from build123d import *

# Parameters (mm, degrees)
SKETCH_R     = 5.5
PAD_DEPTH    = 2
PAD001_DEPTH = 3.6


with BuildPart() as part:
    # Sketch → Pad (new body)
    with BuildSketch(Plane.XY):
        Circle(SKETCH_R)
    extrude(amount=PAD_DEPTH)

    # Sketch001 (on Face3 of Pad) → Pad001 (join)
    with BuildSketch(Plane.XY.offset(2)):
        with BuildLine():
            ThreePointArc((3.122117, 3.720795), (-2.7, 0), (3.122117, -3.720795))
            Line((3.122117, -3.720795), (3.400681, -4.322658))
            ThreePointArc((3.400681, 4.322658), (-5.5, 0), (3.400681, -4.322658))
            Line((3.122117, 3.720795), (3.400681, 4.322658))
        make_face()
    extrude(amount=PAD001_DEPTH)


solid = part.part
Model file for the job. Use its own axes, mm. Coordinates: 2 decimals unless noted, no trailing zeros. Loops run counter-clockwise (first coordinate to the right, second up) from the corner with the lowest first, then second, coordinate; pieces in that order, holes last. Notation, with made-up numbers: (35, -0.5) -> (80, -0.5) arc R35 ccw to (80, 33.5) -> close; hole circle Ø1 at (-11, 59). An arc over 180 degrees is marked (long way). Use one line per item in the form item = value. Start each with the question number.
(1) Probe probe 1 along Z at (x, y) = (-2.5, -0.5); probe 2 along Y at (x, z) = (1.25, 4.4); probe 3 along Y at (x, z) = (1.4, 4.7). List the from-to ranges inside material, lowest first. Write a range as from..to.
(2) Flat gauge pins, fed straight in: pin 1 (4 mm diameter, centred on x = 1, y = 0, fed in from +Z); pin 2 (1 mm diameter, centred on y = -3.5, z = 5, fed in from +X); pin 3 (1 mm diameter, centred on y = -1, z = 2.5, fed in from -X). Where does each tip first touch, or does it go through?
(3) Cut at D-D on y = -1.75. Give the cut face in (x, z).
(4) Cut at C-C on x = -2. Give the cut face in (y, z), and give its area (3 significant figures).
(5) Pull direction X, two halves, no side cores. Call faces 1 (the cylindrical face through (-2.7, 0.1, 3.8)), 2 (the flat face through (-3, 0, 5.6)): pulls with the +X half, pulls with the -X half, needs draft (parallel to the pull), parting line crosses it, or undercut.
(6) Cut at A-A on y = 0. Give the cut face in (x, z).
(7) Cut at B-B on z = 1.25. Give the cut face in (x, y).
Values:
q1.probe_1 = 0..2
q1.probe_2 = -5.36..-4.1, 4.1..5.36
q1.probe_3 = -5.32..-4.1, 4.1..5.32
q2.pin_1 = 2
q2.pin_2 = 3.25
q2.pin_3 = -5.48
q3.outline = (-5.21, 0) -> (5.21, 0) -> (5.21, 2) -> (-2.31, 2) -> (-2.31, 5.6) -> (-5.21, 5.6) -> close
q4.outline = (-5.12, 0) -> (5.12, 0) -> (5.12, 5.6) -> (2.29, 5.6) -> (2.29, 2) -> (-2.29, 2) -> (-2.29, 5.6) -> (-5.12, 5.6) -> close
q4.area = 40.9 mm2
q5.face_1 = undercut
q5.face_2 = needs draft
q6.outline = (-5.5, 0) -> (5.5, 0) -> (5.5, 2) -> (-2.7, 2) -> (-2.7, 5.6) -> (-5.5, 5.6) -> close
q7.outline = circle Ø11 at (0, 0)
